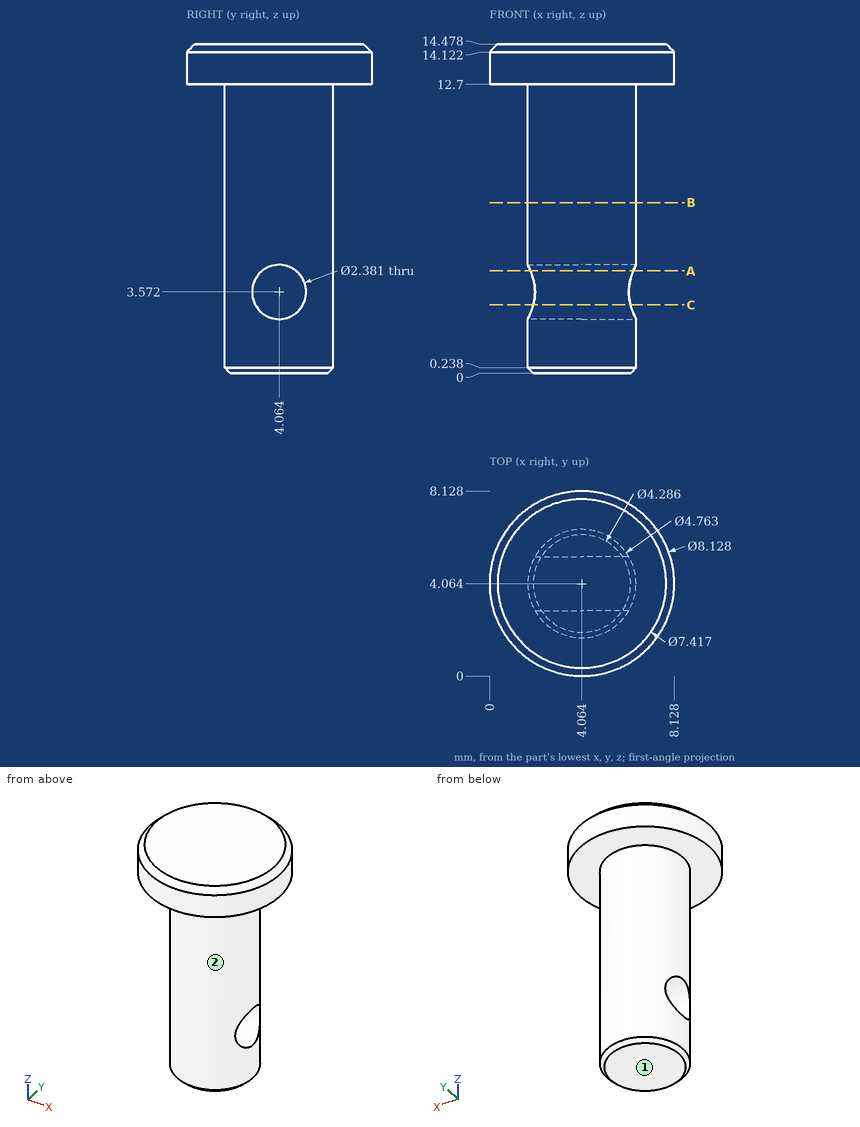
Verification items for this drawing (mm, ordinates from the low corner). A direction names the side the tool comes from. Give positions to 0.01 mm unless a question says otherwise; leave off trailing zeros. Write each loop counter-clockwise with the first axis right and the second up, starting at its lowest first coordinate (ties: lowest second). Pieces come first, ordered by that corner, then holes. Notation, with made-up numbers: (9, 73.25) -> (47, 73.25) arc R7 cw to (47, 86.25) -> close; hole circle Ø7 at (-37.5, -14). An arc over 180 degrees is marked (long way). Write item = value, one per line.
Item 1: Gauge pin test, flat ends, axial feed: pin 1 (1.4 mm diameter, centred on y = 4.06, z = 3.57, fed in from -X); pin 2 (2 mm diameter, centred on y = 5, z = 9.5, fed in from +X) (1 decimal); pin 3 (2.5 mm diameter, centred on y = 4.06, z = 3.57, fed in from -X). Record the tip position at first contact, or that the pin passes through.
Output:
pin_1 = through
pin_2 = 6.4
pin_3 = 1.68
Item 2: Scan lines: probe 1 along X at (y, z) = (4, 11.25) (1 decimal); probe 2 along Y at (x, z) = (5, 3.5) (1 decimal); probe 3 along Z at (x, y) = (7, 6). Record each from-to range of solid material in increasing order. Write a range as from..to.
Output:
probe_1 = 1.7..6.4
probe_2 = 1.9..2.9, 5.3..6.3
probe_3 = 12.7..14.48
Item 3: Sectioned sample at B-B on z = 7.5. Record the boundary of the cut face in (x, y) (1 decimal).
Output:
outline = circle Ø4.8 at (4.1, 4.1)
Item 4: Sectioned sample at C-C on z = 3. Record the boundary of the cut face in (x, y) (1 decimal).
Output:
outline = (1.9, 3) arc R2.4 ccw to (6.2, 3) -> close; (1.9, 5.1) -> (6.2, 5.1) arc R2.4 ccw to start
Item 5: Tool access check on the marked faces 1 and 2. Record the directions out of +Z, -Z, +X, -X, +Y, -Y that give a thin tool (end or side, any length) a straight path to the whole face; none if there is none.
Output:
face_1 = -Z, +X, -X, +Y, -Y
face_2 = -Z
Item 6: Sectioned sample at A-A on z = 4.5. Record the boundary of the cut face in (x, y) (1 decimal), and give its area (3 significant figures).
Output:
outline = (1.8, 3.3) arc R2.4 ccw to (6.3, 3.3) -> close; (1.8, 4.8) -> (6.3, 4.8) arc R2.4 ccw to start
area = 10.8 mm^2
